from build123d import *

# Parameters (mm, degrees)
SKETCH1_W           = 173
SKETCH1_H           = 100
SKETCH1_R           = 3.5
SKETCH1_R_2         = 1.5
SKETCH1_R_3         = 2.5
SKETCH1_R_4         = 2
BOSS_EXTRUDE1_DEPTH = 5


with BuildPart() as part:
    # Sketch1 → Boss-Extrude1 (new body)
    with BuildSketch(Plane(origin=(0, 0, 0), x_dir=(1, 0, 0), z_dir=(0, 1, 0))):
        with Locations((0, -31.8)):
            Rectangle(SKETCH1_W, SKETCH1_H)
        Circle(SKETCH1_R, mode=Mode.SUBTRACT)
        with Locations((-8.5, 0)):
            Circle(SKETCH1_R_2, mode=Mode.SUBTRACT)
        with Locations((8.5, 0)):
            Circle(SKETCH1_R_2, mode=Mode.SUBTRACT)
        with Locations((-30, -10.8)):
            Circle(SKETCH1_R_3, mode=Mode.SUBTRACT)
        with Locations((-30, -52.8)):
            Circle(SKETCH1_R_3, mode=Mode.SUBTRACT)
        with Locations((30, -52.8)):
            Circle(SKETCH1_R_3, mode=Mode.SUBTRACT)
        with Locations((30, -10.8)):
            Circle(SKETCH1_R_3, mode=Mode.SUBTRACT)
        with Locations((63.5, -23.8)):
            Circle(SKETCH1_R_4, mode=Mode.SUBTRACT)
        with Locations((79.5, -23.8)):
            Circle(SKETCH1_R_4, mode=Mode.SUBTRACT)
        with Locations((79.5, -39.8)):
            Circle(SKETCH1_R_4, mode=Mode.SUBTRACT)
        with Locations((63.5, -39.8)):
            Circle(SKETCH1_R_4, mode=Mode.SUBTRACT)
        with Locations((-63.5, -39.8)):
            Circle(SKETCH1_R_4, mode=Mode.SUBTRACT)
        with Locations((-79.5, -39.8)):
            Circle(SKETCH1_R_4, mode=Mode.SUBTRACT)
        with Locations((-79.5, -23.8)):
            Circle(SKETCH1_R_4, mode=Mode.SUBTRACT)
        with Locations((-63.5, -23.8)):
            Circle(SKETCH1_R_4, mode=Mode.SUBTRACT)
    extrude(amount=BOSS_EXTRUDE1_DEPTH)


solid = part.part
Could you check a few things on this model? Use its own coordinates, in mm. Give positions to 0.01 mm unless a question says otherwise; leave off trailing zeros. Order: outer loops, then holes, each group sorted by start corner. A loop starts at its lowest first (then second) coordinate and runs counter-clockwise, first axis right, second up. Notation, with made-up numbers: (53, -15.75) - (72, -15.75) arc R24 cw to (72, -4.75) - close; hole circle Ø1 at (83, -39). An arc over 180 degrees is marked (long way). One line per item, written item: value. Start each with the question number.
1. Imagine slicing it at C-C on z = 10.8. List the corners of the cut face in (x, y) for me.
2. If I drill on probe 1 along X at (y, z) = (3.3, 23.8); probe 2 along Z at (x, y) = (63.5, 3.65); probe 3 along Z at (x, y) = (31, 4.4), over which ranges is the centre line in solid material (lowest first)?
3. For P1, Ø3, axis at x = 79.5, z = 39.8, coming from the -Y side; P2, Ø6, axis at x = 30, z = 10.8, coming from the -Y side, each with a flat end and sliding along its axis, tell me the tip position at first contact or that it passes through.
4. Thinking about a two-plate mould opening in X: for faces 1 (the face through (-86.5, 2, 32)), 2 (the face through (-1, 2, 81.8)), 3 (the face through (63.066, 2.465, 25.752)), 4 (the face through (28.16, 2.46, 51.11)), which applies, +X half, -X half, draft (parallel to the pull), parting line (faces both ways), or undercut?
5. Imagine slicing it at A-A on x = -63.5. List the corners of the cut face in (y, z) for me.
6. Imagine slicing it at B-B on x = 0. List the corners of the cut face in (y, z) for me, plus the area to 3 significant figures.
7. Imagine slicing it at D-D on z = 39.8. List the corners of the cut face in (x, y) for me, plus the area to 3 significant figures.
Values:
1. outline: (-86.5, 0) - (-32.5, 0) - (-32.5, 5) - (-86.5, 5) - close; (-27.5, 0) - (27.5, 0) - (27.5, 5) - (-27.5, 5) - close; (32.5, 0) - (86.5, 0) - (86.5, 5) - (32.5, 5) - close
2. probe 1: -86.5 to -81.5, -77.5 to -65.5, -61.5 to 61.5, 65.5 to 77.5, 81.5 to 86.5
2. probe 2: -18.2 to 21.8, 25.8 to 37.8, 41.8 to 81.8
2. probe 3: -18.2 to 8.51, 13.09 to 50.51, 55.09 to 81.8
3. P1: through
3. P2: y = 0
4. face 1: -X half
4. face 2: draft
4. face 3: undercut
4. face 4: undercut
5. outline: (0, -18.2) - (5, -18.2) - (5, 21.8) - (0, 21.8) - close; (0, 25.8) - (5, 25.8) - (5, 37.8) - (0, 37.8) - close; (0, 41.8) - (5, 41.8) - (5, 81.8) - (0, 81.8) - close
6. outline: (0, -18.2) - (5, -18.2) - (5, -3.5) - (0, -3.5) - close; (0, 3.5) - (5, 3.5) - (5, 81.8) - (0, 81.8) - close
6. area: 465 mm²
7. outline: (-86.5, 0) - (-81.5, 0) - (-81.5, 5) - (-86.5, 5) - close; (-77.5, 0) - (-65.5, 0) - (-65.5, 5) - (-77.5, 5) - close; (-61.5, 0) - (61.5, 0) - (61.5, 5) - (-61.5, 5) - close; (65.5, 0) - (77.5, 0) - (77.5, 5) - (65.5, 5) - close; (81.5, 0) - (86.5, 0) - (86.5, 5) - (81.5, 5) - close
7. area: 785 mm²
